Answer from the drawing. Dimensions are ordinates in mm from the lowest x, y and z of the part. A direction names the side the tool comes from. Round coordinates to 2 decimals unless told otherwise and drop trailing zeros. Order: outer loops, then holes, each group sorted by start corner. A loop starts at its lowest first (then second) coordinate and runs counter-clockwise, first axis right, second up. Notation, with made-up numbers: (55.5, 34.25) -> (78.5, 34.25) arc R20 ccw to (78.5, 46.25) -> close; hole circle Ø5 at (-16.75, -36.5). An arc over 180 degrees is marked (long way). Use a Markdown table: item, result. Add a question column.
Item 1: A cutting plane is placed at D-D, the plane z = 17.5. Determine the outline of the cut face in (x, y), plus the area to 3 significant figures.
Item 2: A cutting plane is placed at A-A, the plane z = 10.5. Determine the outline of the cut face in (x, y).
Item 3: A tool of negligible diameter and unlimited length cuts with its end or side. For the marked faces 1 and 2, from which of +Z, -Z, +X, -X, +Y, -Y can it reach the whole face along a straight path? Write none if from no direction.
Item 4: For a pull along Y with two mould halves and no side action, classify the marked faces 3, 4, 5 and 6 as +Y half, -Y half, draft (parallel to the pull), parting line (faces both ways), or undercut.
Item 5: Find the intervals of material crossed by L1, parallel to Z at x = 10.5, y = 5.75; L2, parallel to Z at x = 10.5, y = 2.2; L3, parallel to X at y = 3.75, z = 6.5, in increasing order. Write a range as [from, to].
Item 6: Flat-ended cylindrical pins translate along their axes: P1, Ø3, axis at x = 12, y = 5.5, coming from the -Z side; P2, Ø4, axis at x = 7, y = 2, coming from the +Z side; P3, Ø3, axis at y = 1.5, z = 7, coming from the +X side. Find the tip coordinate at first contact, or state that the pin passes through.
Item 7: A cutting plane is placed at C-C, the plane x = 10.5. Determine the outline of the cut face in (y, z).
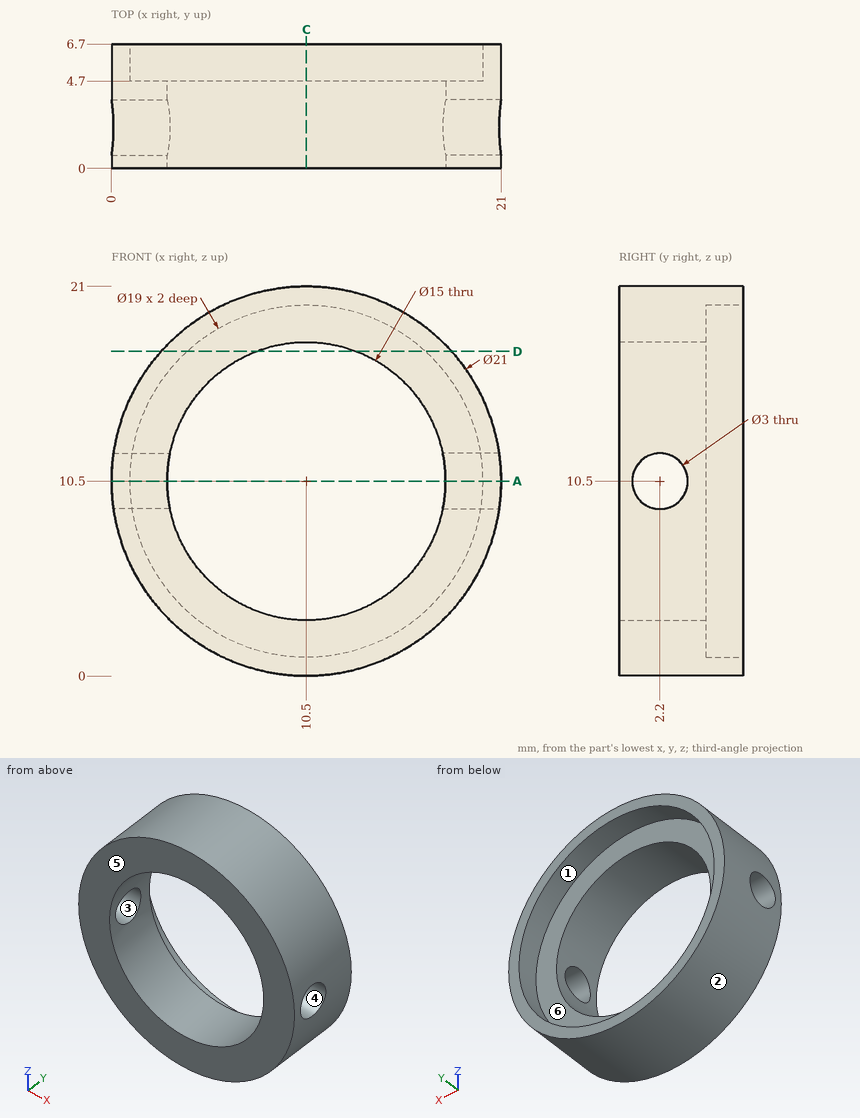
Reported:
| question | item | result |
|---|---|---|
| 1 | outline | (2.67, 0) -> (7.81, 0) -> (7.81, 4.7) -> (4.08, 4.7) -> (4.08, 6.7) -> (2.67, 6.7) -> close; (13.19, 0) -> (18.33, 0) -> (18.33, 6.7) -> (16.92, 6.7) -> (16.92, 4.7) -> (13.19, 4.7) -> close |
| 1 | area | 53.9 mm² |
| 2 | outline | (0, 0) -> (3, 0) -> (3, 0.7) -> (0, 0.7) -> close; (0, 3.7) -> (3, 3.7) -> (3, 4.7) -> (1, 4.7) -> (1, 6.7) -> (0, 6.7) -> close; (18, 0) -> (21, 0) -> (21, 0.7) -> (18, 0.7) -> close; (18, 3.7) -> (21, 3.7) -> (21, 6.7) -> (20, 6.7) -> (20, 4.7) -> (18, 4.7) -> close |
| 3 | face 1 | +Y |
| 3 | face 2 | +Y, -Y |
| 4 | face 3 | undercut |
| 4 | face 4 | undercut |
| 4 | face 5 | -Y half |
| 4 | face 6 | +Y half |
| 5 | L1 | [0, 1], [20, 21] |
| 5 | L2 | [0, 3], [18, 21] |
| 5 | L3 | [0.79, 4.16], [16.84, 20.21] |
| 6 | P1 | z = 0 |
| 6 | P2 | z = 20.89 |
| 6 | P3 | x = 20.81 |
| 7 | outline | (0, 0) -> (6.7, 0) -> (6.7, 1) -> (4.7, 1) -> (4.7, 3) -> (0, 3) -> close; (0, 18) -> (4.7, 18) -> (4.7, 20) -> (6.7, 20) -> (6.7, 21) -> (0, 21) -> close |
